Design review of the part built by this model. Coordinates are the model's own, in mm. A direction names the side the tool comes from. Coordinates: 2 decimals unless noted, no trailing zeros. Loops run counter-clockwise (first coordinate to the right, second up) from the corner with the lowest first, then second, coordinate; pieces in that order, holes last. Notation, with made-up numbers: (9, 70.25) -> (39, 70.25) arc R34 ccw to (39, 103.25) -> close; hole circle Ø10 at (64.25, 73.25). An arc over 180 degrees is marked (long way). One line per item, written item: value. Start each with the question number.
1. Insertion check: pin 1 (4 mm diameter, centred on x = 4.5, y = 2, fed in from -Z); pin 2 (1.5 mm diameter, centred on x = 1, y = -2, fed in from -Z); pin 3 (5 mm diameter, centred on y = 1.5, z = -36, fed in from -X); pin 4 (3 mm diameter, centred on y = 0.5, z = -45.5, fed in from -X). Each pin has a flat end and moves straight along its axis. Give the tip position at first contact, or say it passes through.
2. Draft analysis for pull direction Z (two halves, no side actions). For faces 4 (the flat face through (2.5, -1, -15)), 5 (the cylindrical face through (3.845, -3.388, -48.727)), 6 (the flat face through (1, -4.5, -23)), state which applies: pulls with the +Z half, pulls with the -Z half, needs draft (parallel to the pull), parting line crosses it, or undercut.
3. Add section C-C on z = -36. Write out the cut boundary in (x, y).
4. For probe 1 along Y at (x, z) = (7.4, -46); probe 2 along Z at (x, y) = (3.75, 1.5); probe 3 along Y at (x, z) = (3.2, 0), list the stretches that pass through material, from the lowest coordinate up.
5. Machinability: for faces 1 (the cylindrical face through (0.74, -0.462, -42.853)), 2 (the flat face through (6.3, 2, -45)), 3 (the cylindrical face through (3.955, 2.127, -43.212)), which of the approach directions +Z, -Z, +X, -X, +Y, -Y give a long, thin tool a straight path to every point of the face, cutting with its end or side? Answer none if there is none.
6. Add section B-B on y = -2.25. Write out the cut boundary in (x, z), plus the area to 3 significant figures.
```python
from build123d import *

# Parameters (mm, degrees)
SKETCH_1_R               = 4.5
SKETCH_1_W               = 49.9
SKETCH_1_H               = 7.8
EXTRUDE_1_DEPTH          = 2.5
EXTRUDE_START            = 2.5
SKETCH_1_6_R             = 1.8
SKETCH_1_6_R_2           = 0.25
EXTRUDE_3_DEPTH          = 1.5
SKETCH_1_5_W             = 7.8
SKETCH_1_5_H             = 7.8
EXTRUDE_2_DEPTH          = 7.8
SKETCH_1_7_R             = 2.5
CUT_EXTRUDE_1_DEPTH      = 51.706015422
SKETCH_1_8_R             = 3.15
SKETCH_1_8_R_2           = 2.5
CUT_EXTRUDE_2_DEPTH      = 1.5
CUT_EXTRUDE_START        = 6.3
SKETCH_1_9_R             = 3.15
SKETCH_1_9_R_2           = 2.5
CUT_EXTRUDE_3_DEPTH      = 1.5
SKETCH_2_W               = 0.191868154
SKETCH_2_H               = 2
SKETCH_2_W_2             = 37.6
CUT_EXTRUDE_4_DEPTH      = 51.706015422
FILLET_1_R               = 3.9
CUT_EXTRUDE_5_DEPTH      = 52.59021225
CUT_EXTRUDE_5_DEPTH_BACK = 52.59021225
SKETCH_3_W               = 77.270537225
SKETCH_3_H               = 10.975298688


with BuildPart() as part:
    # 草图1 → 凸台-拉伸1 (new body)
    with BuildSketch(Plane(origin=(0, 0, 0), x_dir=(0, 0, -1), z_dir=(1, 0, 0))):
        Circle(SKETCH_1_R)
        with Locations((24.95, -0.6)):
            Rectangle(SKETCH_1_W, SKETCH_1_H)
    extrude(amount=EXTRUDE_1_DEPTH)

    # 草图1<6> → 凸台-拉伸3 (add)
    with BuildSketch(Plane(origin=(0, 0, 0), x_dir=(0, 0, -1), z_dir=(1, 0, 0)).offset(EXTRUDE_START)):
        Circle(SKETCH_1_6_R)
        Circle(SKETCH_1_6_R_2, mode=Mode.SUBTRACT)
    extrude(amount=EXTRUDE_3_DEPTH)

    # 草图1<5> → 凸台-拉伸2 (add)
    with BuildSketch(Plane(origin=(0, 0, 0), x_dir=(0, 0, -1), z_dir=(1, 0, 0))):
        with Locations((46, -0.6)):
            Rectangle(SKETCH_1_5_W, SKETCH_1_5_H)
    extrude(amount=EXTRUDE_2_DEPTH)

    # 草图1<7> → 切除-拉伸1 (cut, through all)
    with BuildSketch(Plane(origin=(0, 0, 0), x_dir=(0, 0, -1), z_dir=(1, 0, 0))):
        with Locations((46, -0.6)):
            Circle(SKETCH_1_7_R)
    extrude(amount=CUT_EXTRUDE_1_DEPTH, mode=Mode.SUBTRACT)

    # 草图1<8> → 切除-拉伸2 (cut)
    with BuildSketch(Plane(origin=(0, 0, 0), x_dir=(0, 0, -1), z_dir=(1, 0, 0))):
        with Locations((46, -0.6)):
            Circle(SKETCH_1_8_R)
        with Locations((46, -0.6)):
            Circle(SKETCH_1_8_R_2, mode=Mode.SUBTRACT)
    extrude(amount=CUT_EXTRUDE_2_DEPTH, mode=Mode.SUBTRACT)

    # 草图1<9> → 切除-拉伸3 (cut)
    with BuildSketch(Plane(origin=(0, 0, 0), x_dir=(0, 0, -1), z_dir=(1, 0, 0)).offset(CUT_EXTRUDE_START)):
        with Locations((46, -0.6)):
            Circle(SKETCH_1_9_R)
        with Locations((46, -0.6)):
            Circle(SKETCH_1_9_R_2, mode=Mode.SUBTRACT)
    extrude(amount=CUT_EXTRUDE_3_DEPTH, mode=Mode.SUBTRACT)

    # 草图2 → 切除-拉伸4 (cut, through all)
    with BuildSketch(Plane.ZY):
        with BuildLine():
            Line((-3.059411708, 3.3), (-4.308131846, 3.3))
            Line((-4.308131846, 3.3), (-4.308131846, 1.3))
            ThreePointArc((-4.308131846, 1.3), (-3.817089795, 2.383238447), (-3.059411708, 3.3))
        make_face()
        with Locations((-4.404065923, 2.3)):
            Rectangle(SKETCH_2_W, SKETCH_2_H)
        with Locations((-23.3, 2.3)):
            Rectangle(SKETCH_2_W_2, SKETCH_2_H)
    extrude(amount=-CUT_EXTRUDE_4_DEPTH, mode=Mode.SUBTRACT)

    # 圆角1
    fillet_1_edges = [part.edges().sort_by_distance(p)[0] for p in [
        (1.25, 1.3, -4.308131846),
    ]]
    fillet(fillet_1_edges, radius=FILLET_1_R)
    fillet_1_2_edges = [part.edges().sort_by_distance(p)[0] for p in [
        (3.9, -4.5, -49.9),
        (3.9, 3.3, -49.9),
        (5.15, -4.5, -42.1),
        (3.9, 3.3, -42.1),
    ]]
    fillet(fillet_1_2_edges, radius=FILLET_1_R - 0.0001)  # a hair under: the kernel refuses the full size


with BuildPart() as body_2:
    # 镜向2: mirrored copy
    add(part.part.mirror(Plane.ZY.offset(1)))

    # 草图3 → 切除-拉伸5 (cut, two sides: drawn at the far end of the back side and taken through both)
    with BuildSketch(Plane(origin=(-4.5, 0, 0), x_dir=(0, 0, 1), z_dir=(0, -1, 0)).offset(-CUT_EXTRUDE_5_DEPTH_BACK)):
        with Locations((-16.91889565, 1.946720459)):
            Rectangle(SKETCH_3_W, SKETCH_3_H)
    extrude(amount=CUT_EXTRUDE_5_DEPTH + CUT_EXTRUDE_5_DEPTH_BACK, mode=Mode.SUBTRACT)


solid = part.part
```
Worked answers:
1. pin 1: stops at z = -49.85
1. pin 2: stops at z = -49.85
1. pin 3: stops at x = 0
1. pin 4: stops at x = 1.5
2. face 4: undercut
2. face 5: pulls with the -Z half
2. face 6: needs draft
3. outline: (0, -4.5) -> (2.5, -4.5) -> (2.5, 1.3) -> (0, 1.3) -> close
4. probe 1: y = -4.5 to -3.75, 2.55 to 3.3
4. probe 2: z = -49.29 to -47.36, -44.64 to -42.71, -0.99 to 0.99
4. probe 3: y = -1.8 to -0.25, 0.25 to 1.8
5. face 1: -X
5. face 2: +X
5. face 3: +X, +Y
6. outline: (0, -49.53) -> (7.8, -49.53) -> (7.8, -48.68) -> (6.3, -48.68) -> (6.3, -47.88) -> (1.5, -47.88) -> (1.5, -48.68) -> (0, -48.68) -> close; (0, -43.32) -> (1.5, -43.32) -> (1.5, -44.12) -> (6.3, -44.12) -> (6.3, -43.32) -> (7.8, -43.32) -> (7.8, -42.47) -> (2.5, -42.47) -> (2.5, 3.9) -> (0, 3.9) -> close
6. area: 137 mm²
